Geometry: final body of the model. Coordinates: model frame, mm. A direction names the side the tool comes from. Round coordinates to 2 decimals unless told otherwise and drop trailing zeros. Write each question's results on one line, items separated by ' | '.
from build123d import *

# Parameters (mm, degrees)
F0_R     = 10
F1_DEPTH = 10
F1_TAPER = -30
F2_R     = 2
F3_W     = 18
F3_H     = 37.5
F4_DEPTH = 4


with BuildPart() as f1:
    # F0 (on Top) → F1 (new body)
    with BuildSketch(Plane.XY):
        Polygon((7.1782154391, 48.9767620725), (0, 55), (-7.1782154391, 48.9767620725), (-15.8771324027, 9.1666666667), (-46.0042278695, -18.2718641122), (-47.6313972081, -27.5), (-38.8260124304, -30.7048979604), (0, -18.3333333333), (38.8260124304, -30.7048979604), (47.6313972081, -27.5), (46.0042278695, -18.2718641122), (15.8771324027, 9.1666666667), align=None)
        Circle(F0_R, mode=Mode.SUBTRACT)
        Circle(F0_R)
    extrude(amount=F1_DEPTH, taper=F1_TAPER)

    # F2
    f2_edges = [f1.edges().sort_by_distance(p)[0] for p in [
        (0, 58.768386, 5),
        (9.788193, 50.555117, 5),
        (-9.788193, 50.555117, 5),
        (48.676112, -16.800735, 5),
        (50.894915, -29.384193, 5),
        (38.887919, -33.754382, 5),
        (-48.676112, -16.800735, 5),
        (-50.894915, -29.384193, 5),
        (-38.887919, -33.754382, 5),
    ]]
    fillet(f2_edges, radius=F2_R)

    # F3 (on face) → F4 (cut)
    with BuildSketch(Plane.XY.offset(10)):
        with Locations((0, 33.75)):
            Rectangle(F3_W, F3_H)
    extrude(amount=-F4_DEPTH, mode=Mode.SUBTRACT)


solid = f1.part
Q1. Ray query, line 1 along X through (y, z) = (40, 6.75); line 2 along Z through (x, y) = (-5, 36.5); line 3 along Y through (x, z) = (7.5, 7.25). Return the intervals inside material, ascending.
Answer block:
line 1: -13.13 to -9, 9 to 13.13 | line 2: 0 to 6 | line 3: -25.12 to 15, 52.5 to 54.17
Q2. Pin query (flat end, axial travel): pin 1 (1.2 mm diameter, centred on y = 37.5, z = 8, fed in from -X); pin 2 (12 mm diameter, centred on x = -23, y = 26, fed in from +Z); pin 3 (1.5 mm diameter, centred on y = -14.5, z = 8, fed in from +X); pin 4 (2 mm diameter, centred on x = -4.5, z = 7, fed in from -Y). Return the tip coordinate at first contact, or that it passes through.
Answer block:
pin 1: x = -14.79 | pin 2: z = 10 | pin 3: x = 49.77 | pin 4: y = -24.69
Q3. Access query for faces 3 (the flat face through (9, 33, 8)), 4 (the flat face through (-3, -2, 10)). Directions: +Z, -Z, +X, -X, +Y, -Y. A direction counts if a zero-diameter tool reaches every point of the face in a straight line with its end or side. Return the directions, or none.
Answer block:
face 3: +Z | face 4: +Z, +X, -X, +Y, -Y
Q4. Mould query, pull axis X, two halves, no side actions, for faces 1 (the flat face through (-1, -2, 0)), 2 (the flat face through (0, 52.5, 8)). Classes: pulls with the +X half, pulls with the -X half, needs draft (parallel to the pull), parting line crosses it, or undercut.
Answer block:
face 1: needs draft | face 2: undercut
